from build123d import *

# Parameters (mm, degrees)
BOSS_EXTRUDE1_DEPTH = 3
SKETCH4_R           = 4
CUT_EXTRUDE1_DEPTH  = 10


with BuildPart() as part:
    # Sketch3 → Boss-Extrude1 (new body)
    with BuildSketch(Plane(origin=(0, 0, 0), x_dir=(1, 0, 0), z_dir=(0, 1, 0))):
        with BuildLine():
            Line((-150, 100), (-200, 100))
            Line((-200, 100), (-200, 167.359909647))
            ThreePointArc((-200, 167.359909647), (0, 250), (200, 167.359909647))
            Line((200, 167.359909647), (200, 100))
            Line((200, 100), (150, 100))
            Line((150, 100), (150, -100))
            Line((150, -100), (200, -100))
            Line((200, -100), (200, -167.359909647))
            ThreePointArc((200, -167.359909647), (0, -250), (-200, -167.359909647))
            Line((-200, -167.359909647), (-200, -100))
            Line((-200, -100), (-150, -100))
            Line((-150, -100), (-150, 100))
        make_face()
    extrude(amount=BOSS_EXTRUDE1_DEPTH)

    # Sketch4 → Cut-Extrude1 (cut)
    with BuildSketch(Plane(origin=(0, 3, 0), x_dir=(1, 0, 0), z_dir=(0, 1, 0))):
        with Locations(Location((-150, 167.359909647, 0), (0, 0, 270))):
            Circle(SKETCH4_R)
        with Locations(Location((150, 167.359909647, 0), (0, 0, 270))):
            Circle(SKETCH4_R)
        with Locations(Location((150, -167.359909647, 0), (0, 0, 270))):
            Circle(SKETCH4_R)
        with Locations(Location((-150, -167.359909647, 0), (0, 0, 270))):
            Circle(SKETCH4_R)
    extrude(amount=-CUT_EXTRUDE1_DEPTH, mode=Mode.SUBTRACT)


solid = part.part
Read the model definition and answer for the solid it produces. Units are mm, in the model's axes. Coordinates: 2 decimals unless noted, no trailing zeros. Loops run counter-clockwise (first coordinate to the right, second up) from the corner with the lowest first, then second, coordinate; pieces in that order, holes last. Notation, with made-up numbers: (-16, 65) - (14, 65) arc R20 cw to (14, 81) - close; hole circle Ø5 at (13.25, 29.5). An arc over 180 degrees is marked (long way). Answer in a Markdown table with one row per item.
Q1. Find section A-A on x = -165. Write down the section's boundary in (y, z).
Here are the results:
| item | result |
|---|---|
| outline | (0, -197) - (3, -197) - (3, -100) - (0, -100) - close; (0, 100) - (3, 100) - (3, 197) - (0, 197) - close |
Q2. Find section C-C on x = 116.5. Write down the section's boundary in (y, z), plus the area to 3 significant figures.
Here are the results:
| item | result |
|---|---|
| outline | (0, -224.94) - (3, -224.94) - (3, 224.94) - (0, 224.94) - close |
| area | 1,350 mm^2 |
Q3. Given P1, Ø1, axis at y = 2.5, z = -17, coming from the +X side; P2, Ø1.5, axis at x = 181, y = 1.5, coming from the -Z side; P3, Ø0.9, axis at y = 1, z = -41.5, coming from the -X side, each flat-ended and moving along its own axis, determine where each tip first touches the part or whether it passes through.
Here are the results:
| item | result |
|---|---|
| P1 | stops at x = 150 |
| P2 | stops at z = -185.27 |
| P3 | stops at x = -150 |
Q4. Find section B-B on y = 1.15. Write down the section's boundary in (x, z).
Here are the results:
| item | result |
|---|---|
| outline | (-200, -167.36) arc R283.33 ccw to (200, -167.36) - (200, -100) - (150, -100) - (150, 100) - (200, 100) - (200, 167.36) arc R283.33 ccw to (-200, 167.36) - (-200, 100) - (-150, 100) - (-150, -100) - (-200, -100) - close; hole circle Ø8 at (-150, -167.36); hole circle Ø8 at (-150, 167.36); hole circle Ø8 at (150, -167.36); hole circle Ø8 at (150, 167.36) |
Q5. Straight lines are drawn through the part: line 1 along X through (y, z) = (1.3, 9); line 2 along Z through (x, y) = (-168, 2.2); line 3 along Z through (x, y) = (170, 1.85). For each, find the intervals that lie inside material, in ascending order. Write a range as [from, to].
Here are the results:
| item | result |
|---|---|
| line 1 | x = [-150, 150] |
| line 2 | z = [-194.82, -100], [100, 194.82] |
| line 3 | z = [-193.33, -100], [100, 193.33] |
